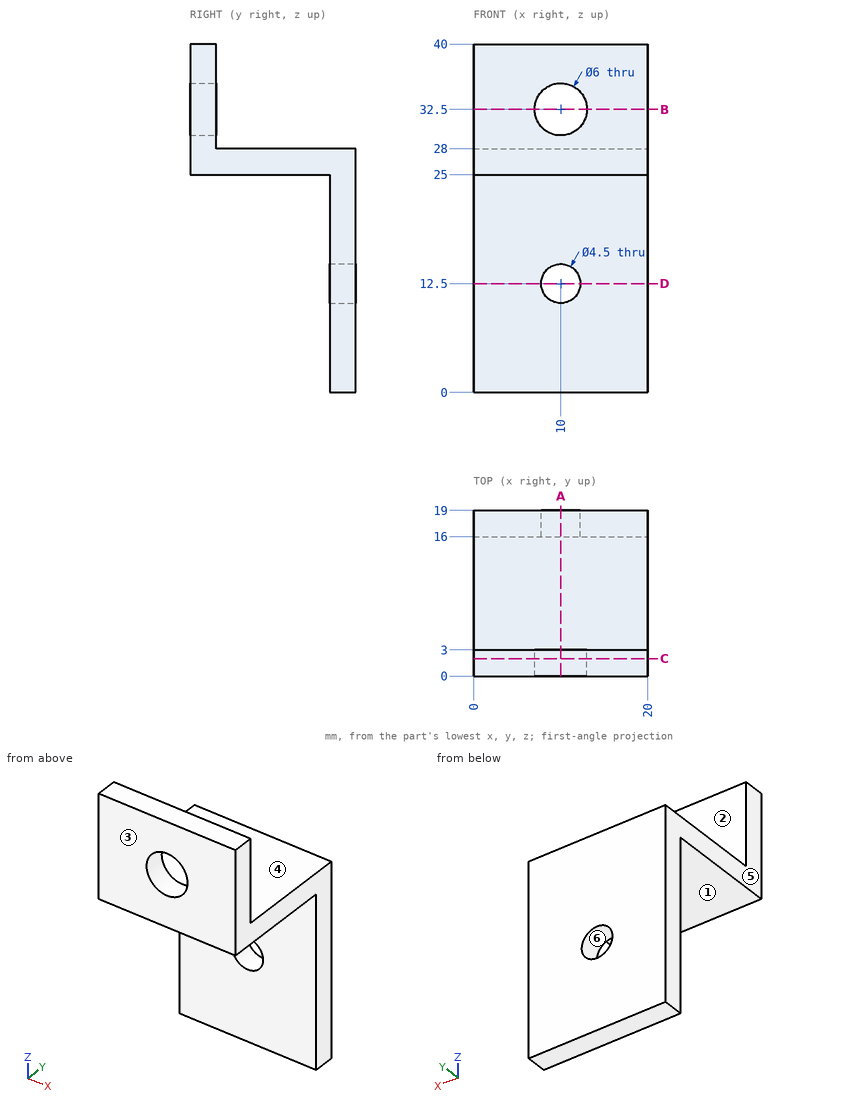
Check sheet for the drawn part. Datum: minimum x, y, z corner. Units: mm. A direction names the side the tool comes from. Round coordinates to 2 decimals unless told otherwise and drop trailing zeros. Order: outer loops, then holes, each group sorted by start corner. A loop starts at its lowest first (then second) coordinate and runs counter-clockwise, first axis right, second up.
1) Section check B-B (z = 32.5). Record the boundary of the cut face in (x, y), and give its area (3 significant figures).
2) Section check A-A (x = 10). Record the boundary of the cut face in (y, z).
3) Section check C-C (y = 2). Record the boundary of the cut face in (x, z).
4) Scan lines: line 1 (Z direction, x = 10, y = 1.4); line 2 (Z direction, x = 10, y = 17.9); line 3 (Y direction, x = 4, z = 10.5). Record each from-to range of solid material in increasing order.
5) Section check D-D (z = 12.5). Record the boundary of the cut face in (x, y).
6) Tool access check on the marked faces 1, 2 and 3. Record the directions out of +Z, -Z, +X, -X, +Y, -Y that give a thin tool (end or side, any length) a straight path to the whole face; none if there is none.
7) Mould release check, pull along Z, two halves, no side actions. Record for the marked faces 4, 5 and 6: +Z half, -Z half, draft (parallel to the pull), parting line (faces both ways), or undercut.
8) Go/stop test with flat-tipped pins: pin 1 Ø1 at (x, z) = (7, 9) entering from -Y; pin 2 Ø8 at (y, z) = (14, 31) entering from +X; pin 3 Ø1.5 at (x, y) = (2.5, 13.5) entering from -Z; pin 4 Ø1.5 at (x, y) = (17.5, 8) entering from +Z. Record where each tip stops, or that it passes through.
Result:
1. outline: (0, 0) - (7, 0) - (7, 3) - (0, 3) - close; (13, 0) - (20, 0) - (20, 3) - (13, 3) - close
1. area: 42.0 mm2
2. outline: (0, 25) - (16, 25) - (16, 14.75) - (19, 14.75) - (19, 28) - (3, 28) - (3, 29.5) - (0, 29.5) - close; (0, 35.5) - (3, 35.5) - (3, 40) - (0, 40) - close; (16, 0) - (19, 0) - (19, 10.25) - (16, 10.25) - close
3. outline: (0, 25) - (20, 25) - (20, 40) - (0, 40) - close; hole circle Ø6 at (10, 32.5)
4. line 1: z = 25 to 29.5, 35.5 to 40
4. line 2: z = 0 to 10.25, 14.75 to 28
4. line 3: y = 16 to 19
5. outline: (0, 16) - (7.75, 16) - (7.75, 19) - (0, 19) - close; (12.25, 16) - (20, 16) - (20, 19) - (12.25, 19) - close
6. face 1: -Z, +X, -X, -Y
6. face 2: +Z, +X, -X, +Y
6. face 3: +Z, -Z, +X, -X, -Y
7. face 4: +Z half
7. face 5: draft
7. face 6: undercut
8. pin 1: stops at y = 16
8. pin 2: stops at x = 20
8. pin 3: stops at z = 25
8. pin 4: stops at z = 28
